```python
from build123d import *

# Parameters (mm, degrees)
F1_DEPTH  = 12.7
F3_D      = 2.9464
F5_D      = 6.35
F6_W      = 6.35
F6_H      = 6.35
F7_DEPTH  = 31.751
F8_DEPTH  = 31.751
F9_R      = 2.778125
F10_DEPTH = 3.175
F13_D     = 1.778
F13_DEPTH = 6.35


with BuildPart() as f1:
    # F0 (on Top) → F1 (new body)
    with BuildSketch(Plane.XY):
        Polygon((0, 19.05), (0, 0), (31.75, 0), (31.75, 19.05), (31.75, 50.8), (25.4, 50.8), (25.4, 19.05), (6.35, 19.05), (6.35, 50.8), (0, 50.8), align=None)
    extrude(amount=F1_DEPTH)

    # F3 (through all)
    with Locations(Plane.XY.offset(12.7)):
        with Locations((3.175, 15.875), (3.175, 3.175), (28.575, 15.875), (28.575, 3.175)):
            Hole(F3_D / 2)

    # F5 (through all)
    with Locations(Plane.YZ.offset(31.75)):
        with Locations((25.4, 6.35), (44.45, 6.35), (34.925, 6.35)):
            Hole(F5_D / 2)

    # F6 (on face) → F7 (cut, through all)
    with BuildSketch(Plane.YZ.offset(31.75)):
        with Locations((34.925, 9.525)):
            Rectangle(F6_W, F6_H)
    extrude(amount=-F7_DEPTH, mode=Mode.SUBTRACT)

    # F6 (on face) → F8 (cut, through all)
    with BuildSketch(Plane.YZ.offset(31.75)):
        with Locations((34.925, 9.525)):
            Rectangle(F6_W, F6_H)
    extrude(amount=-F8_DEPTH, mode=Mode.SUBTRACT)

    # F9 (on face) → F10 (cut)
    with BuildSketch(Plane.XY.offset(12.7)):
        with Locations((3.175, 3.175)):
            Circle(F9_R)
        with Locations((3.175, 15.875)):
            Circle(F9_R)
        with Locations((28.575, 3.175)):
            Circle(F9_R)
        with Locations((28.575, 15.875)):
            Circle(F9_R)
    extrude(amount=-F10_DEPTH, mode=Mode.SUBTRACT)

    # F13
    with Locations(Plane.XY.offset(12.7)):
        with Locations((3.175, 25.4), (3.175, 44.45), (28.575, 25.4), (28.575, 44.45)):
            Hole(F13_D / 2, depth=F13_DEPTH)


solid = f1.part
```
The model under review builds one solid part; all positions refer to its coordinate system, in mm. A direction names the side the tool comes from. Round coordinates to 2 decimals unless told otherwise and drop trailing zeros. Loops run counter-clockwise (first coordinate to the right, second up) from the corner with the lowest first, then second, coordinate; pieces in that order, holes last.
Item 1: Take a section at C-C (z = 5). Give the number of separate pieces and of enclosed holes in the cut face, then the cut area to 3 significant figures.
Determined:
separate pieces: 7
enclosed holes: 4
area: 762 mm2
Item 2: Take a section at D-D (x = 8). Write out the cut boundary in (y, z).
Determined:
outline: (0, 0) - (19.05, 0) - (19.05, 12.7) - (0, 12.7) - close
Item 3: Mouldability with a two-part tool opening along Z and no side actions: class faces 1 (the face through (30, 2, 9.525)), 2 (the face through (3.131, 23.935, 3.533)), 3 (the face through (29, 50.8, 6)) as released by +Z, released by -Z, zero draft, split by the parting line, or undercut.
Determined:
face 1: released by +Z
face 2: undercut
face 3: zero draft
Item 4: Take a section at B-B (y = 30). Write out the cut boundary in (x, z), then the cut area to 3 significant figures.
Determined:
outline: (0, 0) - (6.35, 0) - (6.35, 12.7) - (0, 12.7) - close; (25.4, 0) - (31.75, 0) - (31.75, 12.7) - (25.4, 12.7) - close
area: 161 mm2
Item 5: Take a section at A-A (y = 44.45). Write out the cut boundary in (x, z) (3 decimals), then the cut area to 3 significant figures.
Determined:
outline: (0, 0) - (6.35, 0) - (6.35, 3.175) - (0, 3.175) - close; (0, 9.525) - (2.286, 9.525) - (2.286, 12.7) - (0, 12.7) - close; (4.064, 9.525) - (6.35, 9.525) - (6.35, 12.7) - (4.064, 12.7) - close; (25.4, 0) - (31.75, 0) - (31.75, 3.175) - (25.4, 3.175) - close; (25.4, 9.525) - (27.686, 9.525) - (27.686, 12.7) - (25.4, 12.7) - close; (29.464, 9.525) - (31.75, 9.525) - (31.75, 12.7) - (29.464, 12.7) - close
area: 69.4 mm2
Item 6: Clearance check with flat-ended pins moving along their axes: pin 1 Ø1.1 at (x, y) = (28.575, 25.4) entering from +Z; pin 2 Ø3.5 at (x, y) = (28.575, 3.175) entering from +Z (3 decimals); pin 3 Ø5 at (x, z) = (17, 7.5) entering from +Y; pin 4 Ø1.8 at (x, y) = (28.575, 15.875) entering from -Z. State where each tip first meets the part, or that it passes through.
Determined:
pin 1: stops at z = 3.22
pin 2: stops at z = 9.525
pin 3: stops at y = 19.05
pin 4: passes through
Item 7: For line 1 (X direction, y = 25.4, z = 10.1); line 2 (X direction, y = 20, z = 2.25); line 3 (X direction, y = 3.5, z = 11), list the stretches that pass through material, from the lowest coordinate up.
Determined:
line 1: x = 0 to 2.29, 4.06 to 6.35, 25.4 to 27.69, 29.46 to 31.75
line 2: x = 0 to 6.35, 25.4 to 31.75
line 3: x = 0 to 0.42, 5.93 to 25.82, 31.33 to 31.75
Item 8: For faces 4 (the face through (28.894, 1.737, 4.696)), 5 (the face through (3.88, 43.91, 11.03)), 6 (the face through (6.35, 31, 6)), list the 3-axis set-ups (+Z, -Z, +X, -X, +Y, -Y) from which the entire face can be reached by the end or side of a thin tool; tool diameter is ignored.
Determined:
face 4: +Z, -Z
face 5: +Z
face 6: +Z, -Z, +Y
